Source: three-view drawing plus pictorial views. Frame: mm from the lowest corner of the part. Give positions to 0.01 mm unless a question says otherwise; leave off trailing zeros. Loops run counter-clockwise (first coordinate to the right, second up) from the corner with the lowest first, then second, coordinate; pieces in that order, holes last. Notation, with made-up numbers: (23, 23.25) - (55, 23.25) arc R14 cw to (55, 42.25) - close; hole circle Ø11 at (42.5, -33.5). An arc over 180 degrees is marked (long way). Put each result on its own line as item: value.
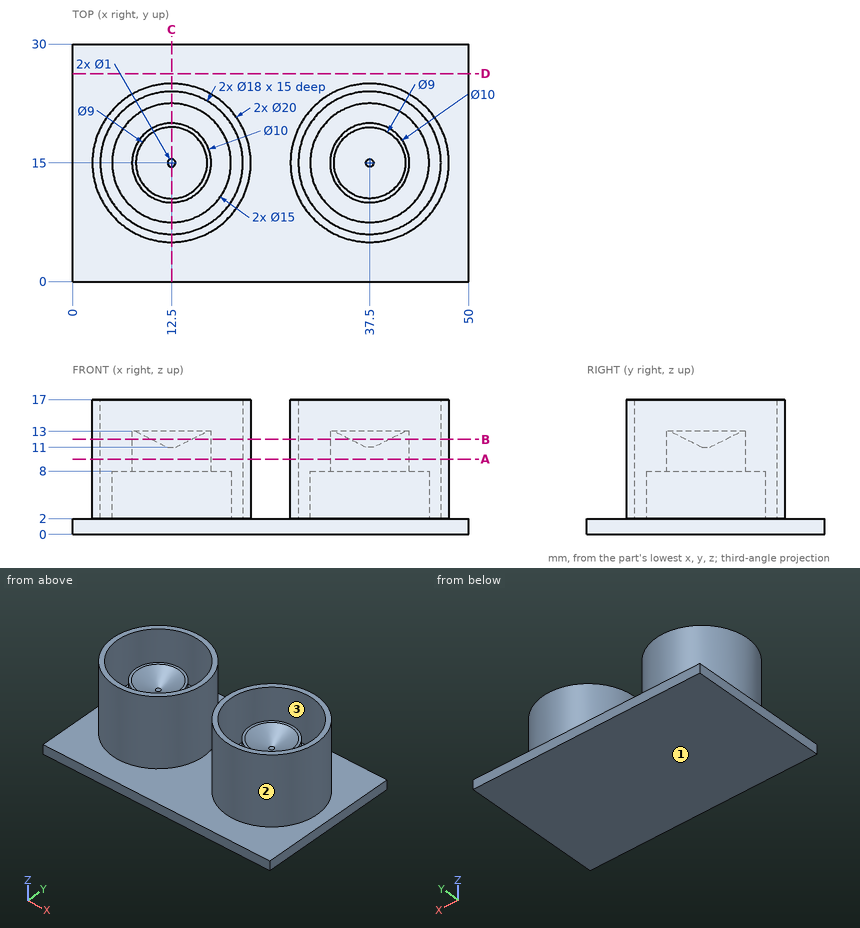
1) Material intervals for line 1 along Y through (x, z) = (37.5, 9); line 2 along Y through (x, z) = (43.5, 3.5); line 3 along X through (y, z) = (23.25, 15.5), sorted ascending. Write a range as [from, to].
Check result:
line 1: [5, 6], [10, 20], [24, 25]
line 2: [7, 8.29], [10.5, 19.5], [21.71, 23]
line 3: [6.85, 8.9], [16.1, 18.15], [31.85, 33.9], [41.1, 43.15]
2) Pin query (flat end, axial travel): P1, Ø5, axis at x = 30.5, z = 11.5, coming from the -Y side; P2, Ø4, axis at x = 28.5, y = 3.5, coming from the +Z side; P3, Ø8, axis at x = 14.5, y = 15, coming from the +Z side. Return the tip coordinate at first contact, or that it passes through.
Check result:
P1: y = 6.07
P2: z = 2
P3: z = 13
3) Section query A-A, the plane z = 9.5. Output: boundary loops of the cut face in (x, y), plus the area to 3 significant figures.
Check result:
outline: circle Ø20 at (12.5, 15); circle Ø10 at (12.5, 15); circle Ø20 at (37.5, 15); circle Ø10 at (37.5, 15); hole circle Ø18 at (12.5, 15); hole circle Ø18 at (37.5, 15)
area: 276 mm²
4) Section query C-C, the plane x = 12.5. Output: boundary loops of the cut face in (y, z).
Check result:
outline: (0, 0) - (30, 0) - (30, 2) - (25, 2) - (25, 17) - (24, 17) - (24, 2) - (22.5, 2) - (22.5, 8) - (20, 8) - (20, 13) - (19.5, 13) - (15.5, 11) - (14.5, 11) - (10.5, 13) - (10, 13) - (10, 8) - (7.5, 8) - (7.5, 2) - (6, 2) - (6, 17) - (5, 17) - (5, 2) - (0, 2) - close
5) Section query B-B, the plane z = 12. Output: boundary loops of the cut face in (x, y), plus the area to 3 significant figures.
Check result:
outline: circle Ø20 at (12.5, 15); circle Ø10 at (12.5, 15); circle Ø20 at (37.5, 15); circle Ø10 at (37.5, 15); hole circle Ø18 at (12.5, 15); hole circle Ø5 at (12.5, 15); hole circle Ø18 at (37.5, 15); hole circle Ø5 at (37.5, 15)
area: 237 mm²
6) Mould query, pull axis X, two halves, no side actions, for the marked faces 1, 2 and 3. Classes: pulls with the +X half, pulls with the -X half, needs draft (parallel to the pull), parting line crosses it, or undercut.
Check result:
face 1: needs draft
face 2: undercut
face 3: undercut
7) Section query D-D, the plane y = 26.25. Output: boundary loops of the cut face in (x, z), plus the area to 3 significant figures.
Check result:
outline: (0, 0) - (50, 0) - (50, 2) - (0, 2) - close
area: 100 mm²
